For this review, take the finished solid that the model builds, in its own axes (mm). A direction names the side the tool comes from. Round coordinates to 2 decimals unless told otherwise and drop trailing zeros. Write each loop counter-clockwise with the first axis right and the second up, starting at its lowest first coordinate (ties: lowest second). Pieces come first, ordered by that corner, then holes.
from build123d import *

# Parameters (mm, degrees)
SKETCH2_R           = 75
BOSS_EXTRUDE1_DEPTH = 1200
SHELL4_T            = 10
BOSS_EXTRUDE2_START = 75
SKETCH3_R           = 30
BOSS_EXTRUDE2_DEPTH = 18
SKETCH10_R          = 30
BOSS_EXTRUDE3_DEPTH = 95
SKETCH12_R          = 20
BOSS_EXTRUDE4_DEPTH = 75


with BuildPart() as part:
    # Sketch2 → Boss-Extrude1 (new body)
    with BuildSketch(Plane(origin=(0, 0, 0), x_dir=(1, 0, 0), z_dir=(0, 1, 0))):
        Circle(SKETCH2_R)
    extrude(amount=BOSS_EXTRUDE1_DEPTH)

    # Shell4 (no face opened: a closed hollow body)
    add(offset(amount=-SHELL4_T, mode=Mode.PRIVATE), mode=Mode.SUBTRACT)

    # Sketch3 → Boss-Extrude2 (add)
    with BuildSketch(Plane.XY.offset(BOSS_EXTRUDE2_START)):
        with BuildLine():
            Line((0, 450), (150, 450))
            ThreePointArc((150, 450), (189.137774485, 418.260424226), (166.164731025, 373.41173042))
            Line((166.164731025, 373.41173042), (0, 300))
            Line((0, 300), (0, 450))
        make_face()
        with BuildLine():
            Line((0, 999), (0, 849))
            Line((0, 849), (-150, 849))
            ThreePointArc((-150, 849), (-189.137774485, 880.739575774), (-166.164731025, 925.58826958))
            Line((-166.164731025, 925.58826958), (0, 999))
        make_face()
        with BuildLine():
            Line((0, 1000), (0, 1200))
            Line((0, 1200), (175.5, 1265.572478983))
            ThreePointArc((175.5, 1265.572478983), (260.246822056, 1235.64155485), (245.673880023, 1146.953824986))
            Line((245.673880023, 1146.953824986), (75, 1000))
            Line((75, 1000), (0, 1000))
        make_face()
        with Locations((200, 1200)):
            Circle(SKETCH3_R, mode=Mode.SUBTRACT)
    boss_extrude2 = extrude(amount=-BOSS_EXTRUDE2_DEPTH)

    # Mirror11: Boss-Extrude2 across plane
    add(boss_extrude2.mirror(Plane(origin=(0, 0, 0), x_dir=(1, 0, 0), z_dir=(0, 0, -1))))

    # Sketch10 → Boss-Extrude3 (add, symmetric)
    with BuildSketch(Plane.XY):
        with Locations((0, 60)):
            Circle(SKETCH10_R)
    extrude(amount=BOSS_EXTRUDE3_DEPTH, both=True)

    # Sketch12 → Boss-Extrude4 (add, symmetric)
    with BuildSketch(Plane.XY):
        with Locations((150, 410)):
            Circle(SKETCH12_R)
        with Locations((-150, 889)):
            Circle(SKETCH12_R)
    extrude(amount=BOSS_EXTRUDE4_DEPTH, both=True)


solid = part.part
(1) For faces 4 (the face through (161.532, 1074.506, 66.126)), 5 (the face through (107, 1137, -75)), 6 (the face through (107, 1137, 75)), 7 (the face through (-102.708, 953.623, -66.126)), 8 (the face through (16, 1096, 57)), list the 3-axis set-ups (+Z, -Z, +X, -X, +Y, -Y) from which the entire face can be reached by the end or side of a thin tool; tool diameter is ignored.
Geometry check:
face 4: +Z, -Z, +X
face 5: -Z, +X, -X, +Y
face 6: +Z, +X, -X, +Y
face 7: -Z, -X, +Y
face 8: none
(2) We need section A-A, the plane z = 35.5. Give the boundary of the cut face in (x, y), and give its area (3 significant figures).
Geometry check:
outline: circle Ø40 at (-150, 889); (-66.07, 0) - (66.07, 0) - (66.07, 1200) - (-66.07, 1200) - close; circle Ø60 at (0, 60); circle Ø40 at (150, 410); hole (-54.45, 10) - (54.45, 10) - (54.45, 1190) - (-54.45, 1190) - close
area: 35,400 mm2
(3) We need section D-D, the plane y = 60. Give the boundary of the cut face in (x, z).
Geometry check:
outline: (-30, -95) - (30, -95) - (30, -68.74) arc R75 ccw to (30, 68.74) - (30, 95) - (-30, 95) - (-30, 68.74) arc R75 ccw to (-30, -68.74) - close; hole (-30, -57.66) - (-30, 57.66) arc R65 ccw to start; hole (30, -57.66) arc R65 ccw to (30, 57.66) - close
(4) For pin 1 Ø1.5 at (x, y) = (64, 659) entering from -Z; pin 2 Ø1 at (y, z) = (652, -20) entering from +X; pin 3 Ø2.5 at (x, z) = (8.5, 59.5) entering from +Y, all flat-tipped, find the tip position at first contact; note any pin that passes through.
Geometry check:
pin 1: stops at z = -40.3
pin 2: stops at x = 72.42
pin 3: stops at y = 1203.64
(5) We need section C-C, the plane y = 590.5. Give the boundary of the cut face in (x, z), and give its area (3 significant figures).
Geometry check:
outline: circle Ø150 at (0, 0); hole circle Ø130 at (0, 0)
area: 4,400 mm2
(6) We need section B-B, the plane y = 410. Give the boundary of the cut face in (x, z), and give its area (3 significant figures).
Geometry check:
outline: (0, -75) - (190, -75) - (190, -57) - (170, -57) - (170, 57) - (190, 57) - (190, 75) - (0, 75) arc R75 ccw to start; hole (0, -65) - (0, -57) - (31.24, -57) arc R65 ccw to (31.24, 57) - (0, 57) - (0, 65) arc R65 ccw to start; hole (48.74, -57) - (130, -57) - (130, 57) - (48.74, 57) arc R75 cw to start
area: 14,900 mm2
(7) For line 1 along Z through (x, y) = (131, 1051); line 2 along X through (y, z) = (876, 55.5); line 3 along Y through (x, z) = (55, 12.5), list the stretches that pass through material, from the lowest coordinate up.
Geometry check:
line 1: z = -75 to -57, 57 to 75
line 2: x = -165.2 to -134.8, -50.45 to -33.83, 33.83 to 50.45
line 3: y = 0 to 10, 1190 to 1200
(8) Mouldability with a two-part tool opening along Z and no side actions: class faces 1 (the face through (-6.503, 30.713, 0.91)), 2 (the face through (0, 60, -95)), 3 (the face through (161.532, 1074.506, -66.126)) as pulls with the +Z half, pulls with the -Z half, needs draft (parallel to the pull), parting line crosses it, or undercut.
Geometry check:
face 1: undercut
face 2: pulls with the -Z half
face 3: needs draft
